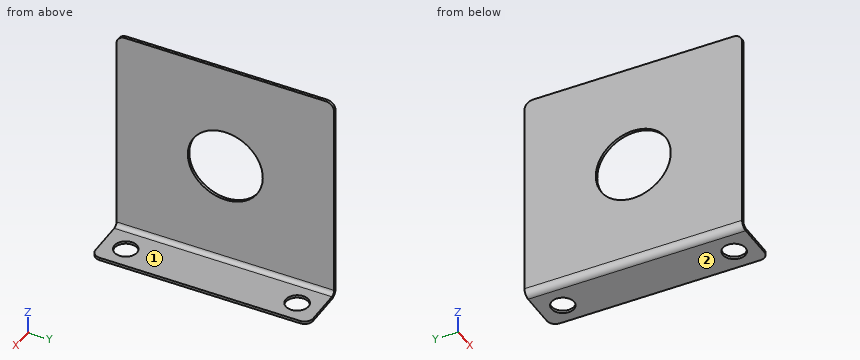
from build123d import *

# Parameters (mm, degrees)
SKETCH1_W                    = 50
SKETCH1_H                    = 50.8
BASE_FLANGE1_DEPTH           = 0.635
SKETCH9_R                    = 8.75
CUT_EXTRUDE1_DEPTH           = 36.644960724
EDGE_FLANGE1_STRIP_W         = 4.54
EDGE_FLANGE1_STRIP_H         = 0.635
EDGE_FLANGE1_STRIP_CUT_DEPTH = 50.8
EDGE_FLANGE1_DEPTH           = 50.8
SKETCH13_R                   = 2.65
CUT_EXTRUDE2_DEPTH           = 57.667684354
FILLET1_R                    = 2


# Sheet-metal steps are written as plain solids
with BuildPart() as part:
    # Sketch1 → Base-Flange1 (new body)
    with BuildSketch(Plane(origin=(0, 0, 0), x_dir=(0, 0, -1), z_dir=(1, 0, 0))):
        Rectangle(SKETCH1_W, SKETCH1_H)
    extrude(amount=-BASE_FLANGE1_DEPTH)

    # Sketch9 → Cut-Extrude1 (cut, through all)
    with BuildSketch(Plane(origin=(0, 0, 0), x_dir=(0, 0, -1), z_dir=(1, 0, 0))):
        Circle(SKETCH9_R)
    extrude(amount=-CUT_EXTRUDE1_DEPTH, mode=Mode.SUBTRACT)

    # Edge-Flange1 strip (across the edge) → Edge-Flange1 strip cut (cut)
    with BuildSketch(Plane(origin=(0, -25.4, -25), x_dir=(0, 0, 1), z_dir=(0, 1, 0))):
        with Locations((-0.635, -0.3175)):
            Rectangle(EDGE_FLANGE1_STRIP_W, EDGE_FLANGE1_STRIP_H)
    extrude(amount=EDGE_FLANGE1_STRIP_CUT_DEPTH, mode=Mode.SUBTRACT)

    # Edge-Flange1 section (across the edge) → Edge-Flange1 (add)
    with BuildSketch(Plane(origin=(0, -25.4, -25), x_dir=(0, 0, 1), z_dir=(0, 1, 0))):
        with BuildLine():
            Line((0, 1), (0, 11.365))
            Line((0, 11.365), (0.635, 11.365))
            Line((0.635, 11.365), (0.635, 1))
            ThreePointArc((0.635, 1), (0.927893219, 0.292893219), (1.635, 0))
            Line((1.635, 0), (1.635, -0.635))
            ThreePointArc((1.635, -0.635), (0.478880413, -0.156119587), (0, 1))
        make_face()
    extrude(amount=EDGE_FLANGE1_DEPTH)

    # Sketch13 → Cut-Extrude2 (cut, through all)
    with BuildSketch(Plane.XY.offset(-24.365)):
        with Locations((6.1825, -20)):
            Circle(SKETCH13_R)
        with Locations((6.1825, 20)):
            Circle(SKETCH13_R)
    extrude(amount=-CUT_EXTRUDE2_DEPTH, mode=Mode.SUBTRACT)

    # Fillet1
    fillet1_edges = [part.edges().sort_by_distance(p)[0] for p in [
        (11.365, -25.4, -24.6825),
        (11.365, 25.4, -24.6825),
        (-0.3175, -25.4, 25),
        (-0.3175, 25.4, 25),
    ]]
    fillet(fillet1_edges, radius=FILLET1_R)


solid = part.part
Here's how the part is built. I have some questions about the finished solid (model axes, mm). Face numbers are marked on the shaded views. A direction names the side the tool comes from. Give positions to 0.01 mm unless a question says otherwise; leave off trailing zeros. Order: outer loops, then holes, each group sorted by start corner. A loop starts at its lowest first (then second) coordinate and runs counter-clockwise, first axis right, second up. Notation, with made-up numbers: (-2.5, 25.25) -> (35.5, 25.25) arc R27 ccw to (35.5, 53.25) -> close; hole circle Ø3 at (-21, 47.25). An arc over 180 degrees is marked (long way). Use a Markdown table: item, result. Add a question column.
Item 1: Imagine slicing it at C-C on x = 8. Please give me the cut outline in (y, z) (3 decimals), plus the area to 3 significant figures.
Item 2: Imagine slicing it at A-A on z = 0. Please give me the cut outline in (x, y) (3 decimals).
Item 3: For the marked faces 1 and 2, which set-ups out of +Z, -Z, +X, -X, +Y, -Y let a thin tool reach every point of the face, with its end or its side?
Item 4: Imagine slicing it at D-D on y = -20. Please give me the cut outline in (x, z) (1 decimal), plus the area to 3 significant figures.
Item 5: Imagine slicing it at B-B on y = 0. Please give me the cut outline in (x, z) (3 decimals), plus the area to 3 significant figures.
Item 6: I need wall thicknesses on line 1 (Z direction, x = 1, y = 10) (3 decimals); line 2 (X direction, y = -0.5, z = 19) (3 decimals); line 3 (Z direction, x = 0.25, y = 21). Which ranges of each line are inside material? Lowest first, please.
Item 7: Will these pins go through, and if not, where does the flat tip stop? pin 1 (4 mm diameter, centred on x = 6.5, y = 5, fed in from +Z) (3 decimals); pin 2 (14.5 mm diameter, centred on y = 5, z = -7.5, fed in from +X); pin 3 (6 mm diameter, centred on y = -0.5, z = 3, fed in from +X).
Data:
| question | item | result |
|---|---|---|
| 1 | outline | (-25.4, -25) -> (-21.929, -25) -> (-21.929, -24.365) -> (-25.4, -24.365) -> close; (-18.071, -25) -> (18.071, -25) -> (18.071, -24.365) -> (-18.071, -24.365) -> close; (21.929, -25) -> (25.4, -25) -> (25.4, -24.365) -> (21.929, -24.365) -> close |
| 1 | area | 27.4 mm² |
| 2 | outline | (-0.635, -25.4) -> (0, -25.4) -> (0, -8.75) -> (-0.635, -8.75) -> close; (-0.635, 8.75) -> (0, 8.75) -> (0, 25.4) -> (-0.635, 25.4) -> close |
| 3 | face 1 | +Z, +X, +Y, -Y |
| 3 | face 2 | -Z, +X, -X, +Y, -Y |
| 4 | outline | (-0.6, -23.4) arc R1.6 ccw to (1, -25) -> (3.5, -25) -> (3.5, -24.4) -> (1, -24.4) arc R1 cw to (0, -23.4) -> (0, 25) -> (-0.6, 25) -> close; (8.8, -25) -> (11.4, -25) -> (11.4, -24.4) -> (8.8, -24.4) -> close |
| 4 | area | 35.2 mm² |
| 5 | outline | (-0.635, -23.365) arc R1.635 ccw to (1, -25) -> (11.365, -25) -> (11.365, -24.365) -> (1, -24.365) arc R1 cw to (0, -23.365) -> (0, -8.75) -> (-0.635, -8.75) -> close; (-0.635, 8.75) -> (0, 8.75) -> (0, 25) -> (-0.635, 25) -> close |
| 5 | area | 27.5 mm² |
| 6 | line 1 | z = -25 to -24.365 |
| 6 | line 2 | x = -0.635 to 0 |
| 6 | line 3 | z = -24.82 to -24.03 |
| 7 | pin 1 | stops at z = -24.365 |
| 7 | pin 2 | stops at x = 0 |
| 7 | pin 3 | passes through |
